Part print with two shaded views. Sizes in mm from the minimum x, y, z corner. A direction names the side the tool comes from. Give positions to 0.01 mm unless a question says otherwise; leave off trailing zeros. Order: outer loops, then holes, each group sorted by start corner. A loop starts at its lowest first (then second) coordinate and runs counter-clockwise, first axis right, second up. Notation, with made-up numbers: (-2.5, 13) - (34.5, 13) arc R20 ccw to (34.5, 35) - close; hole circle Ø6 at (79.5, 6.5). An arc over 180 degrees is marked (long way). Return JSON: item names as keys, results as strings. Group by question number.
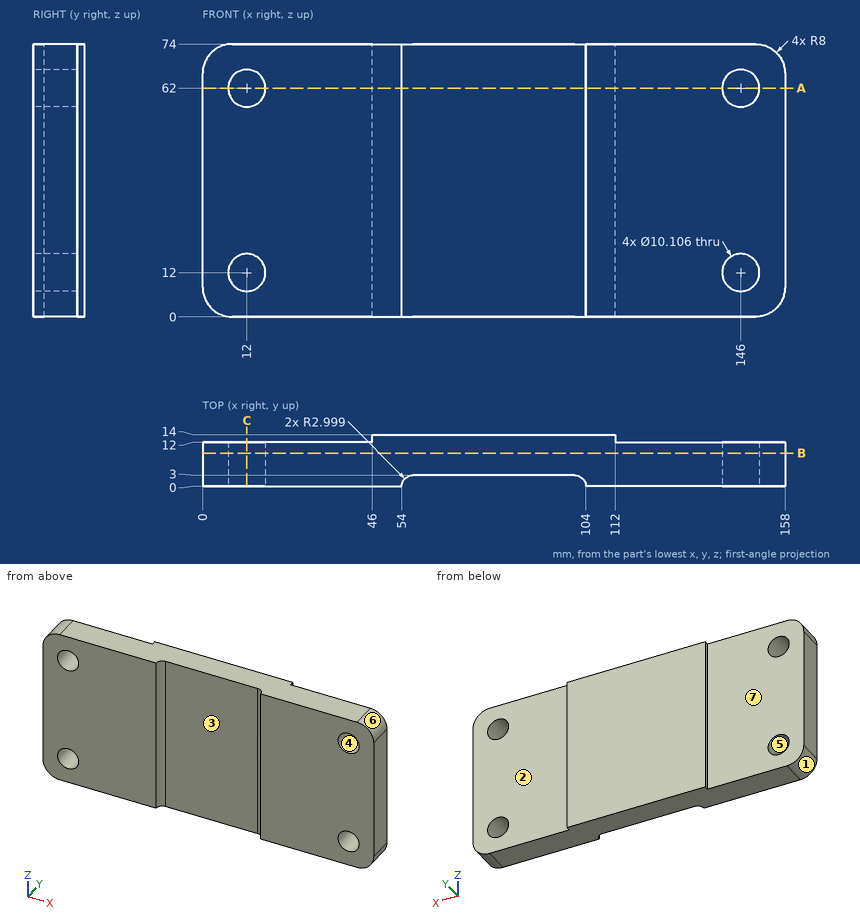
(1) Slice it at A-A (z = 62). State how many separate pieces and enclosed holes the cut face has, and give its area (3 significant figures).
(2) Drill centre lines: L1, parallel to Z at x = 12, y = 5.5; L2, parallel to X at y = 3.75, z = 12; L3, parallel to Y at x = 10.5, z = 70.5. Where is each one in solid material? Low to high.
(3) Drop flat-ended pins along their axis: pin 1 Ø16 at (x, z) = (12, 62) entering from -Y; pin 2 Ø23 at (x, z) = (14, 36.5) entering from +Y; pin 3 Ø1 at (y, z) = (13.5, 45) entering from -X; pin 4 Ø0.6 at (y, z) = (12.5, 28) entering from +X. Give the stop position or say it passes through.
(4) Slice it at B-B (y = 9). Give the cut face in (x, z) (1 decimal), and give its area (3 significant figures).
(5) Pull direction Z, two halves, no side cores. Call the marked faces 4, 5, 6 and 7: released by +Z, released by -Z, zero draft, split by the parting line, or undercut.
(6) Slice it at C-C (x = 12). Give the cut face in (y, z).
(7) 3-axis set-ups, long thin cutter, end or side, ignore diameter. For the marked faces 1, 2 and 3: which of +Z, -Z, +X, -X, +Y, -Y reach the whole face in a straight line?
Result set:
{
 "1": {"separate pieces": "3", "enclosed holes": "0", "area": "1,640 mm²"},
 "2": {"L1": "z = 0 to 6.95, 17.05 to 56.95, 67.05 to 74", "L2": "x = 0 to 6.95, 17.05 to 140.95, 151.05 to 158", "L3": "y = 0 to 12"},
 "3": {"pin 1": "stops at y = 0", "pin 2": "stops at y = 12", "pin 3": "stops at x = 46", "pin 4": "stops at x = 112"},
 "4": {"outline": "(0, 8) arc R8 ccw to (8, 0) - (150, 0) arc R8 ccw to (158, 8) - (158, 66) arc R8 ccw to (150, 74) - (8, 74) arc R8 ccw to (0, 66) - close; hole circle Ø10.1 at (12, 12); hole circle Ø10.1 at (12, 62); hole circle Ø10.1 at (146, 12); hole circle Ø10.1 at (146, 62)", "area": "11,300 mm²"},
 "5": {"face 4": "undercut", "face 5": "undercut", "face 6": "released by +Z", "face 7": "zero draft"},
 "6": {"outline": "(0, 0) - (12, 0) - (12, 6.95) - (0, 6.95) - close; (0, 17.05) - (12, 17.05) - (12, 56.95) - (0, 56.95) - close; (0, 67.05) - (12, 67.05) - (12, 74) - (0, 74) - close"},
 "7": {"face 1": "-Z, -X, +Y, -Y", "face 2": "+Z, -Z, +X, +Y", "face 3": "+Z, -Z, -Y"}
}
